Input: part model. Units: mm. Frame: model coordinates. Face numbers are marked on the shaded views. A direction names the side the tool comes from. Coordinates: 2 decimals unless noted, no trailing zeros. Answer as CSV lines item,"result". Start each with the question number.
Item 1: First-contact query: pin 1 (1 mm diameter, centred on x = -0.5, y = -1, fed in from +Z); pin 2 (1.5 mm diameter, centred on x = 2.5, y = -6, fed in from -Z). Flat tips, straight axial feed; report the tip coordinate or a pass-through.
Item 2: Material intervals for line 1 along X through (y, z) = (-3.25, 0) (3 decimals); line 2 along X through (y, z) = (-5.5, 0); line 3 along Z through (x, y) = (1, -1), sorted ascending.
Item 3: Access query for the marked faces 4 and 5. Directions: +Z, -Z, +X, -X, +Y, -Y. A direction counts if a zero-diameter tool reaches every point of the face in a straight line with its end or side. Return the directions, or none.
Item 4: Draft query along X for the marked faces 1, 2 and 3. Return one class per face: +X half, -X half, draft (parallel to the pull), parting line (faces both ways), or undercut.
from build123d import *

# Parameters (mm, degrees)
EXTRUDE1_DEPTH = 8
SKETCH4_R      = 2.350480947
EXTRUDE2_DEPTH = 11.029476557


with BuildPart() as part:
    # Sketch1 → Extrude1 (new body)
    with BuildSketch(Plane(origin=(0, 0, 0), x_dir=(1, 0, 0), z_dir=(0, 1, 0))):
        Polygon((0, 4.572614132), (-3.96, 2.286307066), (-3.96, -2.286307066), (0, -4.572614132), (3.96, -2.286307066), (3.96, 2.286307066), align=None)
    extrude(amount=-EXTRUDE1_DEPTH)

    # Sketch4 → Extrude2 (cut, through all)
    with BuildSketch(Plane(origin=(0, 0, 0), x_dir=(-1, 0, 0), z_dir=(0, 1, 0))):
        with Locations(Location((0, 0, 0), (0, 0, 90))):
            Circle(SKETCH4_R)
    extrude(amount=-EXTRUDE2_DEPTH, mode=Mode.SUBTRACT)

    # Sketch5 → Cut-Revolve1 (revolve, cut)
    with BuildSketch(Plane.XY):
        Polygon((-3.945, -8), (-4.572614132, -8), (-5.200228264, -8), (-5.200228264, 0), (-4.572614132, 0), (-4.572614132, -0.666666667), (-3.945, -0.666666667), (-3.945, -1.666666667), (-4.555159067, -1.666666667), (-4.548720402, -2.035537527), (-3.945, -2.897739617), (-3.945, -3.266666667), (-4.527230963, -3.266666667), (-4.520792298, -3.635537527), (-3.945, -4.457854151), (-3.945, -4.826781201), (-4.499999063, -4.826781201), (-4.493560398, -5.195652062), (-3.945, -5.9790775), (-3.945, -6.34800455), (-4.47344601, -6.34800455), (-4.467007346, -6.716875411), (-3.945, -7.462379161), align=None)
    revolve(axis=Axis((0, 0, 0), (0, -1, 0)), mode=Mode.SUBTRACT)


solid = part.part
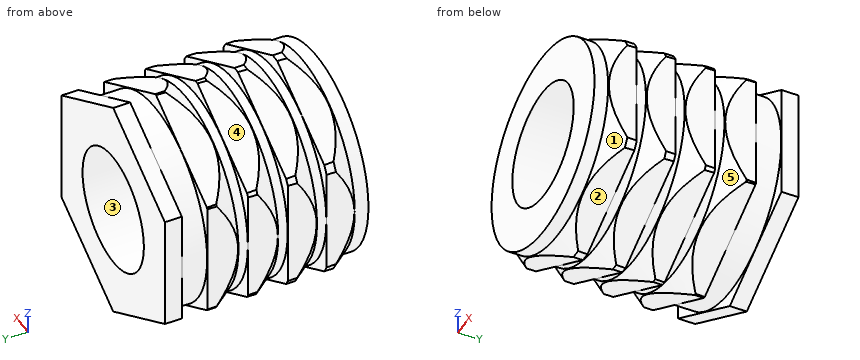
Determined:
1,pin 1,"stops at z = 4.5"
1,pin 2,"stops at z = -3.56"
2,line 1,"x = -3.945 to -2.35, 2.35 to 3.945"
2,line 2,"x = -3.96 to -2.35, 2.35 to 3.96"
2,line 3,"z = -3.82 to -2.13, 2.13 to 3.82"
3,face 4,"+Z, -X, +Y, -Y"
3,face 5,"none"
4,face 1,"parting line"
4,face 2,"+X half"
4,face 3,"undercut"
